Build history of the part. All positions in model axes, mm. A direction names the side the tool comes from. Give positions to 0.01 mm unless a question says otherwise; leave off trailing zeros. Order: outer loops, then holes, each group sorted by start corner. A loop starts at its lowest first (then second) coordinate and runs counter-clockwise, first axis right, second up. Notation, with made-up numbers: M -12,-27 L 33,-27 A25 cw 33,-14 Z; hole C 1.25,-22 d1. An arc over 180 degrees is marked long. One line per item, written item: value.
from build123d import *

# Parameters (mm, degrees)
SKETCH1_W           = 152.4
SKETCH1_H           = 38.1
BOSS_EXTRUDE1_DEPTH = 107.95
SKETCH2_R           = 1.35255
CUT_EXTRUDE1_DEPTH  = 152.4
SKETCH3_R           = 6.477
CUT_EXTRUDE4_DEPTH  = 154.686
SKETCH4_R           = 11.557
CUT_EXTRUDE5_DEPTH  = 2.54
CUT_EXTRUDE6_DEPTH  = 152.4
CHAMFER1_SIZE       = 6.35
FILLET1_R           = 10
FILLET2_R           = 2.54


with BuildPart() as part:
    # Sketch1 → Boss-Extrude1 (new body)
    with BuildSketch(Plane.XY):
        with Locations((-76.2, -19.05)):
            Rectangle(SKETCH1_W, SKETCH1_H)
    extrude(amount=BOSS_EXTRUDE1_DEPTH)

    # Sketch2 → Cut-Extrude1 (cut)
    with BuildSketch(Plane(origin=(0, 0, 0), x_dir=(0, 0, -1), z_dir=(1, 0, 0))):
        with Locations(Location((-73.025, -6.35, 0), (0, 0, 90))):
            Circle(SKETCH2_R)
        with BuildLine():
            ThreePointArc((-52.62245, -25.4), (-53.018602723, -24.443602723), (-53.975, -24.04745))
            Line((-53.975, -24.04745), (-53.975, -26.75255))
            ThreePointArc((-53.975, -26.75255), (-53.018602723, -26.356397277), (-52.62245, -25.4))
        make_face()
        with BuildLine():
            Line((-53.975, -26.75255), (-53.975, -24.04745))
            ThreePointArc((-53.975, -24.04745), (-55.32755, -25.4), (-53.975, -26.75255))
        make_face()
        with Locations(Location((-34.925, -6.35, 0), (0, 0, 90))):
            Circle(SKETCH2_R)
    extrude(amount=-CUT_EXTRUDE1_DEPTH, mode=Mode.SUBTRACT)

    # Sketch3 → Cut-Extrude4 (cut)
    with BuildSketch(Plane(origin=(0, 0, 0), x_dir=(0, 0, -1), z_dir=(1, 0, 0))):
        with Locations(Location((-53.975, -6.5024, 0), (0, 0, 90))):
            Circle(SKETCH3_R)
    extrude(amount=-CUT_EXTRUDE4_DEPTH, mode=Mode.SUBTRACT)

    # Sketch4 → Cut-Extrude5 (cut)
    with BuildSketch(Plane(origin=(0, 0, 0), x_dir=(0, 0, -1), z_dir=(1, 0, 0))):
        with Locations((-53.975, -6.5024)):
            Circle(SKETCH4_R)
    cut_extrude5 = extrude(amount=-CUT_EXTRUDE5_DEPTH, mode=Mode.SUBTRACT)

    # Mirror1: Cut-Extrude5 across plane
    add(cut_extrude5.mirror(Plane(origin=(-76.2, 0, 0), x_dir=(0, 0, 1), z_dir=(1, 0, 0))), mode=Mode.SUBTRACT)

    # Sketch5 → Cut-Extrude6 (cut)
    with BuildSketch(Plane(origin=(0, 0, 0), x_dir=(0, 0, -1), z_dir=(1, 0, 0))):
        with BuildLine():
            Line((-107.95, -9.525), (-79.375, -9.525))
            ThreePointArc((-79.375, -9.525), (-53.975, -30.327663184), (-28.575, -9.525))
            Line((-28.575, -9.525), (0, -9.525))
            Line((0, -9.525), (0, -59.754484856))
            Line((0, -59.754484856), (-107.95, -59.754484856))
            Line((-107.95, -59.754484856), (-107.95, -9.525))
        make_face()
    extrude(amount=-CUT_EXTRUDE6_DEPTH, mode=Mode.SUBTRACT)

    # Chamfer1
    # the kernel refuses this chamfer: 6.35 mm, written as the material it adds along each edge
    with BuildSketch(Plane(origin=(0, -9.525, 79.375), x_dir=(0, -0.9387392646709182, -0.34462819525555927), z_dir=(-1, 0, 0))) as chamfer1_piece_1:
        with BuildLine():
            Line((7.921952063, 0), (-CHAMFER1_SIZE * 0.344628195256, CHAMFER1_SIZE * 0.938739264671))
            Line((-CHAMFER1_SIZE * 0.344628195256, CHAMFER1_SIZE * 0.938739264671), (0, 0))
            ThreePointArc((0, 0), (4.071956682, 0.304341963), (7.921952063, 0))
        make_face()
    extrude(amount=152.4)
    with BuildSketch(Plane(origin=(0, -9.525, 28.575), x_dir=(0, 0, -1), z_dir=(-1, 0, 0))) as chamfer1_piece_2:
        with BuildLine():
            Line((CHAMFER1_SIZE, 0), (-2.730128042, 7.436647454))
            ThreePointArc((-2.730128042, 7.436647454), (-1.117613332, 3.927390442), (0, 0))
            Line((0, 0), (CHAMFER1_SIZE, 0))
        make_face()
    extrude(amount=152.4)

    # Fillet1
    fillet1_edges = [part.edges().sort_by_distance(p)[0] for p in [
        (-76.2, -9.525, 85.725),
        (-76.2, -16.961647454, 31.305128042),
        (-76.2, -16.961647454, 76.644871958),
        (-76.2, -9.525, 22.225),
    ]]
    fillet(fillet1_edges, radius=FILLET1_R)

    # Fillet2
    fillet2_edges = [part.edges().sort_by_distance(p)[0] for p in [
        (-152.4, -4.7625, 107.95),
        (-152.4, -4.7625, 0),
        (0, -4.7625, 0),
        (0, -4.7625, 107.95),
    ]]
    fillet(fillet2_edges, radius=FILLET2_R)


solid = part.part
1) Drill centre lines: probe 1 along Z at (x, y) = (-114, -6); probe 2 along Z at (x, y) = (-55.5, -12); probe 3 along Y at (x, z) = (-105, 6.5) (3 decimals). Where is each one in solid material? Low to high. Write a range as from..to.
Check values:
probe 1: 0..33.62, 36.23..47.52, 60.43..71.72, 74.33..107.95
probe 2: 25.25..50.55, 57.4..82.7
probe 3: -9.525..0
2) Saw through at D-D, the plane z = 86.5. Write the cut outline in (x, y).
Check values:
outline: M -152.4,-9.92 L 0,-9.92 L 0,0 L -152.4,0 Z
3) Tool access for faces 1 (the face through (-75, -9.525, 9)), 2 (the face through (-75, -9.525, 99)), 3 (the face through (-151.148, -18.054, 54.326)), 4 (the face through (-2.54, -13, 52)): list every direction of +Z, -Z, +X, -X, +Y, -Y with a clear straight run to the whole face (end or side of a thin tool).
Check values:
face 1: -Z, +X, -X, -Y
face 2: +Z, +X, -X, -Y
face 3: -X
face 4: +X
4) Saw through at C-C, the plane z = 38. Write the cut outline in (x, y), then the cut area to 3 significant figures.
Check values:
outline: M -152.4,-24.82 L 0,-24.82 L 0,0 L -152.4,0 Z
area: 3,780 mm^2
5) Mould opens along Y. For faces 5 (the face through (0, -19, 55)), 6 (the face through (-1.252, -18.054, 54.326)), 7 (the face through (-77, 0, 65)) say: released by +Y, released by -Y, zero draft, split by the parting line, or undercut.
Check values:
face 5: zero draft
face 6: undercut
face 7: released by +Y
6) Saw through at A-A, the plane z = 51. Write the cut outline in (x, y).
Check values:
outline: M -152.4,-30.16 L 0,-30.16 L 0,-17.67 L -2.54,-17.67 L -2.54,-12.26 L -149.86,-12.26 L -149.86,-17.67 L -152.4,-17.67 Z; M -149.86,-0.75 L -2.54,-0.75 L -2.54,0 L -149.86,0 Z
7) Pin check, flat tips, straight feed: pin 1 (5 mm diameter, centred on x = -56, y = -25, fed in from +Z); pin 2 (1.5 mm diameter, centred on x = -34.5, z = 95, fed in from -Y) (3 decimals); pin 3 (2.5 mm diameter, centred on y = -6.35, z = 73.025, fed in from -X); pin 4 (5 mm diameter, centred on x = -46, z = 78.5, fed in from -Y). Stop position of each tip, or through.
Check values:
pin 1: z = 72.53
pin 2: y = -9.525
pin 3: through
pin 4: y = -18.07
8) Saw through at B-B, the plane x = -46.5. Write the cut outline in (y, z) (3 decimals), then the cut area to 3 significant figures.
Check values:
outline: M -18.247,32.065 A10 cw -15.848,29.945 L -11.789,24.989 A10 cw -9.525,18.653 L -9.525,0 L 0,0 L 0,107.95 L -9.525,107.95 L -9.525,89.297 A10 cw -11.789,82.961 L -15.848,78.005 A10 cw -18.247,75.885 A25.908 ccw Z; hole C -25.4,53.975 d2.705; hole C -6.502,53.975 d12.954; hole C -6.35,34.925 d2.705; hole C -6.35,73.025 d2.705
area: 1,720 mm^2
